Check sheet for the modelled part. Datum: model origin and axes. Units: mm. Round coordinates to 2 decimals unless told otherwise and drop trailing zeros. Write each loop counter-clockwise with the first axis right and the second up, starting at its lowest first coordinate (ties: lowest second). Pieces come first, ordered by that corner, then holes.
Item 1: Material ranges on line 1 (X direction, y = 4.5, z = 6.5); line 2 (X direction, y = 1.5, z = 6.5); line 3 (X direction, y = 2, z = 6.5), recorded low to high.
Item 2: Cross-section at B-B on z = 6.5. Enter the section's corners in (x, y) (3 decimals), plus the area to 3 significant figures.
Item 3: Cross-section at D-D on y = 3.5. Enter the section's corners in (x, z), plus the area to 3 significant figures.
Item 4: Release check for a two-part mould opening along X. For faces 1 (the flat face through (10, 3, 7)), 2 (the flat face through (29, 0, 6)), 3 (the cylindrical face through (25.41, 3.13, 6.18)) record: +X half, -X half, draft (parallel to the pull), parting line (faces both ways), or undercut.
Item 5: Cross-section at C-C on y = 0.75. Enter the section's corners in (x, z).
Item 6: Cross-section at A-A on x = 26.85. Enter the section's corners in (y, z).
from build123d import *

# Parameters (mm, degrees)
SKETCH1_W           = 21
SKETCH1_H           = 13
SKETCH1_R           = 1.4732
BOSS_EXTRUDE1_DEPTH = 6.35
CUT_EXTRUDE1_DEPTH  = 13


with BuildPart() as part:
    # Sketch1 → Boss-Extrude1 (new body)
    with BuildSketch(Plane(origin=(0, 0, 0), x_dir=(1, 0, 0), z_dir=(0, 1, 0))):
        with Locations((20.5, -6.5)):
            Rectangle(SKETCH1_W, SKETCH1_H)
        with Locations(Location((14.15, -6.5, 0), (0, 0, 270))):
            Circle(SKETCH1_R, mode=Mode.SUBTRACT)
        with Locations(Location((26.85, -6.5, 0), (0, 0, 270))):
            Circle(SKETCH1_R, mode=Mode.SUBTRACT)
    extrude(amount=BOSS_EXTRUDE1_DEPTH)

    # Sketch2 → Cut-Extrude1 (cut)
    with BuildSketch(Plane(origin=(0, 0, 0), x_dir=(-1, 0, 0), z_dir=(0, 0, -1))):
        with BuildLine():
            ThreePointArc((-17.39358, 0), (-20.5, 2.518661837), (-23.60642, 0))
            Line((-23.60642, 0), (-17.39358, 0))
        make_face()
        with BuildLine():
            Line((-17.39358, 0), (-23.60642, 0))
            ThreePointArc((-23.60642, 0), (-20.829955679, -3.814146619), (-17.325, -0.656338163))
            ThreePointArc((-17.325, -0.656338163), (-17.342191543, -0.326382484), (-17.39358, 0))
        make_face()
    extrude(amount=-CUT_EXTRUDE1_DEPTH, mode=Mode.SUBTRACT)


solid = part.part
Response values:
1. line 1: x = 10 to 12.68, 15.62 to 25.38, 28.32 to 31
1. line 2: x = 10 to 12.68, 15.62 to 18.17, 22.83 to 25.38, 28.32 to 31
1. line 3: x = 10 to 12.68, 15.62 to 18.76, 22.24 to 25.38, 28.32 to 31
2. outline: (10, 0) - (12.677, 0) - (12.677, 6.35) - (10, 6.35) - close; (15.623, 0) - (17.394, 0) arc R3.175 cw to (23.606, 0) - (25.377, 0) - (25.377, 6.35) - (15.623, 6.35) - close; (28.323, 0) - (31, 0) - (31, 6.35) - (28.323, 6.35) - close
2. area: 84.2 mm2
3. outline: (10, 0) - (31, 0) - (31, 13) - (10, 13) - close; hole circle Ø2.95 at (14.15, 6.5); hole circle Ø2.95 at (26.85, 6.5)
3. area: 259 mm2
4. face 1: -X half
4. face 2: draft
4. face 3: undercut
5. outline: (10, 0) - (17.65, 0) - (17.65, 13) - (10, 13) - close; (23.35, 0) - (31, 0) - (31, 13) - (23.35, 13) - close; hole circle Ø2.95 at (14.15, 6.5); hole circle Ø2.95 at (26.85, 6.5)
6. outline: (0, 0) - (6.35, 0) - (6.35, 5.03) - (0, 5.03) - close; (0, 7.97) - (6.35, 7.97) - (6.35, 13) - (0, 13) - close
